from build123d import *

# Parameters (mm, degrees)
EXTRUDE_1_DEPTH     = 32
SKETCH_3_R          = 1.25
CUT_EXTRUDE_2_DEPTH = 60.464274989
SKETCH_5_R          = 2.2
CUT_EXTRUDE_3_DEPTH = 45.631827209
SKETCH_6_W          = 8.988665833
SKETCH_6_H          = 24
CUT_EXTRUDE_4_DEPTH = 60.464274989


with BuildPart() as part:
    # 草图1 → 凸台-拉伸1 (new body)
    with BuildSketch(Plane.XY):
        Polygon((-22, 0), (22, 0), (22, 24), (20, 24), (20, 2), (-20, 2), (-20, 24), (-22, 24), align=None)
    extrude(amount=EXTRUDE_1_DEPTH)

    # 草图3 → 切除-拉伸2 (cut, through all)
    with BuildSketch(Plane(origin=(22, 0, 0), x_dir=(0, 0, -1), z_dir=(1, 0, 0))):
        with Locations((-3.5, 20.5)):
            Circle(SKETCH_3_R)
        with Locations((-18.5, 20.5)):
            Circle(SKETCH_3_R)
        with Locations((-11, 20.5)):
            Circle(SKETCH_3_R)
        with Locations(Location((-3.5, 5.5, 0), (0, 0, 270))):
            Circle(SKETCH_3_R)
        with Locations(Location((-11, 5.5, 0), (0, 0, 270))):
            Circle(SKETCH_3_R)
        with Locations(Location((-18.5, 5.5, 0), (0, 0, 270))):
            Circle(SKETCH_3_R)
        with Locations((-18.5, 13)):
            Circle(SKETCH_3_R)
    extrude(amount=-CUT_EXTRUDE_2_DEPTH, mode=Mode.SUBTRACT)

    # 草图5 → 切除-拉伸3 (cut, through all)
    with BuildSketch(Plane(origin=(0, 2, 0), x_dir=(1, 0, 0), z_dir=(0, 1, 0))):
        with Locations(Location((-15, -27, 0), (0, 0, 270))):
            Circle(SKETCH_5_R)
        with Locations(Location((15, -27, 0), (0, 0, 90))):
            Circle(SKETCH_5_R)
    extrude(amount=-CUT_EXTRUDE_3_DEPTH, mode=Mode.SUBTRACT)

    # 草图6 → 切除-拉伸4 (cut, through all)
    with BuildSketch(Plane(origin=(22, 0, 0), x_dir=(0, 0, -1), z_dir=(1, 0, 0))):
        with Locations((-27.505667084, 12)):
            Rectangle(SKETCH_6_W, SKETCH_6_H)
    extrude(amount=-CUT_EXTRUDE_4_DEPTH, mode=Mode.SUBTRACT)


solid = part.part
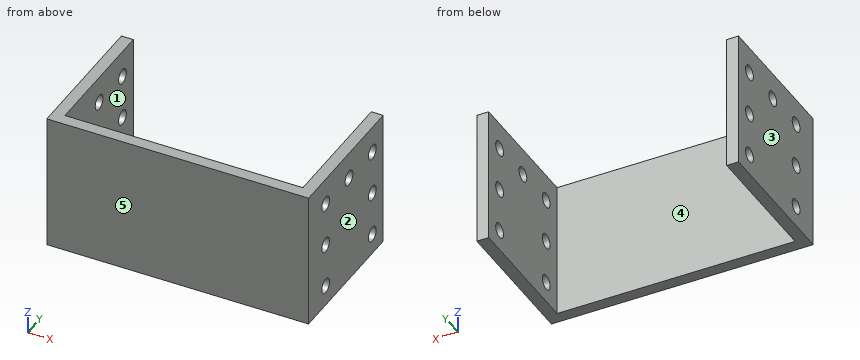
The listing builds one solid part. Answer for the finished solid, in the listing's coordinates (mm). Face numbers are marked on the shaded views. A direction names the side the tool comes from. Give positions to 0.01 mm unless a question says otherwise; leave off trailing zeros. Loops run counter-clockwise (first coordinate to the right, second up) from the corner with the lowest first, then second, coordinate; pieces in that order, holes last.
Item 1: A tool of negligible diameter and unlimited length cuts with its end or side. For the marked faces 4 and 5, from which of +Z, -Z, +X, -X, +Y, -Y can it reach the whole face along a straight path? Write none if from no direction.
Derived:
face 4: +Z, -Z, +Y
face 5: +Z, -Z, +X, -X, -Y
Item 2: Find the intervals of material crossed by line 1 along Z through (x, y) = (21.65, 5.5); line 2 along Y through (x, z) = (20.95, 11); line 3 along Y through (x, z) = (21.4, 18.5), in increasing order.
Derived:
line 1: z = 0 to 2.25, 4.75 to 9.75, 12.25 to 17.25, 19.75 to 23.01
line 2: y = 0 to 4.25, 6.75 to 19.25, 21.75 to 24
line 3: y = 0 to 4.25, 6.75 to 11.75, 14.25 to 19.25, 21.75 to 24
Item 3: Determine the mould class of the marked faces 1, 2 and 3 for opening direction X: +X half, -X half, draft (parallel to the pull), parting line (faces both ways), or undercut.
Derived:
face 1: undercut
face 2: +X half
face 3: -X half
Item 4: Each of these flat-tipped pins is pushed along its axis until it touches: pin 1 Ø3 at (y, z) = (13, 18.5) entering from +X; pin 2 Ø7 at (x, z) = (8.5, 14) entering from +Y. Where does it stop, or does it pass through?
Derived:
pin 1: stops at x = 22
pin 2: stops at y = 2
Item 5: A cutting plane is placed at B-B (z = 18.5). Give the number of separate pieces and of enclosed holes in the cut face, then the cut area to 3 significant figures.
Derived:
separate pieces: 7
enclosed holes: 0
area: 146 mm2
Item 6: A cutting plane is placed at A-A (z = 3.5). Give the vertices of the cut face in (x, y).
Derived:
outline: (-22, 0) - (22, 0) - (22, 4.25) - (20, 4.25) - (20, 2) - (-20, 2) - (-20, 4.25) - (-22, 4.25) - close; (-22, 6.75) - (-20, 6.75) - (-20, 19.25) - (-22, 19.25) - close; (-22, 21.75) - (-20, 21.75) - (-20, 24) - (-22, 24) - close; (20, 6.75) - (22, 6.75) - (22, 19.25) - (20, 19.25) - close; (20, 21.75) - (22, 21.75) - (22, 24) - (20, 24) - close
Item 7: A cutting plane is placed at C-C (y = 22.75). Give the vertices of the cut face in (x, z), then the cut area to 3 significant figures.
Derived:
outline: (-22, 0) - (-20, 0) - (-20, 23.01) - (-22, 23.01) - close; (20, 0) - (22, 0) - (22, 23.01) - (20, 23.01) - close
area: 92.0 mm2
